Here's how the part is built. I have some questions about the finished solid (model axes, mm). Face numbers are marked on the shaded views. Give positions to 0.01 mm unless a question says otherwise; leave off trailing zeros. Write each loop counter-clockwise with the first axis right and the second up, starting at its lowest first coordinate (ties: lowest second). Pieces come first, ordered by that corner, then holes. Notation, with made-up numbers: (-25.75, 67.5) - (17.25, 67.5) arc R12 ccw to (17.25, 73.5) - close; hole circle Ø2 at (21, 81). An arc over 180 degrees is marked (long way). Use a Markdown table: item, result.
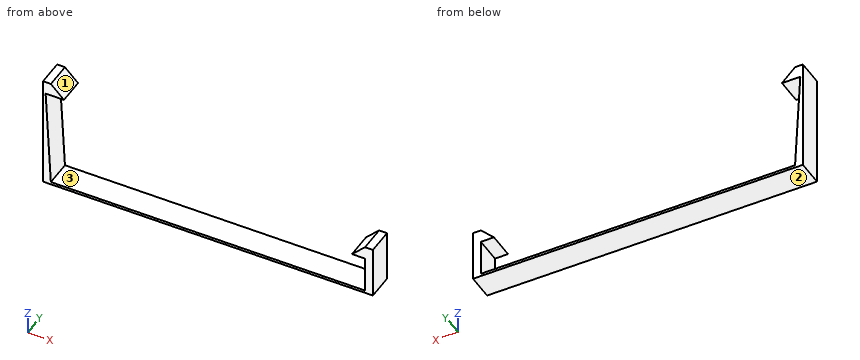
```python
from build123d import *

# Parameters (mm, degrees)
F0_W     = 126
F0_H     = 1
F1_DEPTH = 10
F2_W     = 3
F2_H     = 10
F3_DEPTH = 43
F4_DEPTH = 19
F6_DEPTH = 10
F7_DEPTH = 10
F9_DEPTH = 25


with BuildPart() as f1:
    # F0 (on Front) → F1 (new body)
    with BuildSketch(Plane.XZ):
        with Locations((0, 0.5)):
            Rectangle(F0_W, F0_H)
    extrude(amount=F1_DEPTH)

    # F2 (on face) → F3 (join)
    with BuildSketch(Plane.XY.offset(1)):
        with Locations((-61.5, -5)):
            Rectangle(F2_W, F2_H)
    extrude(amount=F3_DEPTH)

    # F2 (on face) → F4 (join)
    with BuildSketch(Plane.XY.offset(1)):
        with Locations((61.5, -5)):
            Rectangle(F2_W, F2_H)
    extrude(amount=F4_DEPTH)

    # F5 (on face) → F6 (join)
    with BuildSketch(Plane.XZ.offset(10)):
        Polygon((-55, 39), (-60, 44), (-60, 39), align=None)
    extrude(amount=-F6_DEPTH)

    # F5 (on face) → F7 (join)
    with BuildSketch(Plane.XZ.offset(10)):
        Polygon((55, 15), (60, 15), (60, 20), align=None)
    extrude(amount=-F7_DEPTH)

    # F8 (on face) → F9 (cut)
    with BuildSketch(Plane.XZ.offset(10)):
        Polygon((-62, 39), (-60, 1), (-60, 39), align=None)
    extrude(amount=-F9_DEPTH, mode=Mode.SUBTRACT)


solid = f1.part
```
Item 1: If we section it at B-B, the plane y = -5.5: Write out the boundary of the cut face in (x, z), plus the area to 3 significant figures.
Values:
| item | result |
|---|---|
| outline | (-63, 0) - (63, 0) - (63, 20) - (60, 20) - (55, 15) - (60, 15) - (60, 1) - (-60, 1) - (-62, 39) - (-55, 39) - (-60, 44) - (-63, 44) - close |
| area | 299 mm2 |
Item 2: I need wall thicknesses on line 1 along Z through (x, y) = (6, -2.25); line 2 along X through (y, z) = (-7.25, 11); line 3 along Z through (x, y) = (-57, -2). Which ranges of each line are inside material? Lowest first, please. Write a range as [from, to].
Values:
| item | result |
|---|---|
| line 1 | z = [0, 1] |
| line 2 | x = [-63, -60.53], [60, 63] |
| line 3 | z = [0, 1], [39, 41] |
Item 3: Will these pins go through, and if not, where does the flat tip stop? pin 1 Ø1.5 at (x, y) = (61, -2.5) entering from +Z; pin 2 Ø2 at (x, y) = (-4.5, -2) entering from +Z.
Values:
| item | result |
|---|---|
| pin 1 | stops at z = 20 |
| pin 2 | stops at z = 1 |
Item 4: Thinking about a two-plate mould opening in X: for the marked faces 1, 2 and 3, which applies, +X half, -X half, draft (parallel to the pull), parting line (faces both ways), or undercut?
Values:
| item | result |
|---|---|
| face 1 | +X half |
| face 2 | draft |
| face 3 | undercut |
Item 5: If we section it at D-D, the plane z = 31: Write out the boundary of the cut face in (x, y), plus the area to 3 significant figures.
Values:
| item | result |
|---|---|
| outline | (-63, -10) - (-61.58, -10) - (-61.58, 0) - (-63, 0) - close |
| area | 14.2 mm2 |
Item 6: If we section it at C-C, the plane x = 0.5: Write out the boundary of the cut face in (y, z).
Values:
| item | result |
|---|---|
| outline | (-10, 0) - (0, 0) - (0, 1) - (-10, 1) - close |
Item 7: If we section it at A-A, the plane z = 10.5: Write out the boundary of the cut face in (x, y).
Values:
| item | result |
|---|---|
| outline | (-63, -10) - (-60.5, -10) - (-60.5, 0) - (-63, 0) - close; (60, -10) - (63, -10) - (63, 0) - (60, 0) - close |
